```python
from build123d import *

# Parameters (mm, degrees)
BOSS_EXTRUDE1_DEPTH          = 3.175
F_10_CLEARANCE_HOLE1_D       = 4.9784
F_10_0_1935_DIAMETER_HOLE1_D = 4.9149


with BuildPart() as part:
    # Sketch1 → Boss-Extrude1 (new body)
    with BuildSketch(Plane.XY):
        Polygon((-253.5966335, 0), (-266.700000508, 0), (-266.700000508, 63.5), (-254.000000508, 63.5), (-254.000000508, 25.4), (-241.300000508, 12.7), (-203.200000508, 12.7), (-203.200000508, 0), align=None)
    extrude(amount=BOSS_EXTRUDE1_DEPTH)

    # #10 Clearance Hole1 (through all)
    with Locations(Plane.XY.offset(3.175)):
        with Locations((-260.350000508, 6.35), (-260.350000508, 25.4), (-241.300000508, 6.35), (-215.900000508, 6.35)):
            Hole(F_10_CLEARANCE_HOLE1_D / 2)

    # #10 (0.1935) Diameter Hole1 (through all)
    with Locations(Plane.XY.offset(3.175)):
        with Locations((-260.350000508, 50.8)):
            Hole(F_10_0_1935_DIAMETER_HOLE1_D / 2)


solid = part.part
```
Part model, mm, in its own coordinate system. A direction names the side the tool comes from. Give positions to 0.01 mm unless a question says otherwise; leave off trailing zeros. Loops run counter-clockwise (first coordinate to the right, second up) from the corner with the lowest first, then second, coordinate; pieces in that order, holes last. Notation, with made-up numbers: M -6.5,89 L 50.5,89 A20 ccw 50.5,114 Z; hole C -33,27 d9. An arc over 180 degrees is marked long. Return JSON: item names as keys, results as strings.
1) Saw through at C-C, the plane x = -215.9. List the corners of the cut face in (y, z) (3 decimals), then the cut area to 3 significant figures.
Calculated:
{"outline": "M 0,0 L 3.861,0 L 3.861,3.175 L 0,3.175 Z; M 8.839,0 L 12.7,0 L 12.7,3.175 L 8.839,3.175 Z", "area": "24.5 mm2"}
2) Drill centre lines: line 1 (Y direction, x = -260.35, z = 2.4); line 2 (Y direction, x = -215.9, z = 1.75); line 3 (X direction, y = 39.5, z = 0.7). Where is each one in solid material? Low to high.
Calculated:
{"line 1": "y = 0 to 3.86, 8.84 to 22.91, 27.89 to 48.34, 53.26 to 63.5", "line 2": "y = 0 to 3.86, 8.84 to 12.7", "line 3": "x = -266.7 to -254"}
3) Pull direction Y, two halves, no side cores. Call faces 3 (the face through (-259.82, 48.4, 1.57)), 4 (the face through (-203.2, 6, 2)), 5 (the face through (-247.7, 19.1, 1.6)): released by +Y, released by -Y, zero draft, split by the parting line, or undercut.
Calculated:
{"face 3": "undercut", "face 4": "zero draft", "face 5": "released by +Y"}
4) Saw through at B-B, the plane z = 1. List the corners of the cut face in (x, y).
Calculated:
{"outline": "M -266.7,0 L -203.2,0 L -203.2,12.7 L -241.3,12.7 L -254,25.4 L -254,63.5 L -266.7,63.5 Z; hole C -260.35,6.35 d4.98; hole C -260.35,25.4 d4.98; hole C -260.35,50.8 d4.91; hole C -241.3,6.35 d4.98; hole C -215.9,6.35 d4.98"}
5) Flat gauge pins, fed straight in: pin 1 Ø1.6 at (y, z) = (48, 1) entering from +X; pin 2 Ø5.5 at (x, y) = (-241.3, 6.35) entering from +Z (3 decimals); pin 3 Ø3 at (x, y) = (-260.35, 6.35) entering from +Z. Where does each tip first touch, or does it go through?
Calculated:
{"pin 1": "stops at x = -254", "pin 2": "stops at z = 3.175", "pin 3": "passes through"}
6) 3-axis set-ups, long thin cutter, end or side, ignore diameter. For faces 1 (the face through (-238.813, 6.459, 1.565)), 2 (the face through (-223, 12.7, 2)): which of +Z, -Z, +X, -X, +Y, -Y reach the whole face in a straight line?
Calculated:
{"face 1": "+Z, -Z", "face 2": "+Z, -Z, +X, +Y"}
7) Saw through at D-D, the plane x = -230.5. List the corners of the cut face in (y, z) (3 decimals).
Calculated:
{"outline": "M 0,0 L 12.7,0 L 12.7,3.175 L 0,3.175 Z"}
8) Saw through at A-A, the plane y = 50.8. List the corners of the cut face in (x, z) (3 decimals).
Calculated:
{"outline": "M -266.7,0 L -262.807,0 L -262.807,3.175 L -266.7,3.175 Z; M -257.893,0 L -254,0 L -254,3.175 L -257.893,3.175 Z"}
